```python
from build123d import *

# Parameters (mm, degrees)
BOSS_EXTRUDE1_DEPTH = 0.3
SKETCH2_R           = 0.35
CUT_EXTRUDE1_DEPTH  = 0.3
CUT_EXTRUDE2_DEPTH  = 0.1


with BuildPart() as part:
    # Sketch1 → Boss-Extrude1 (new body)
    with BuildSketch(Plane(origin=(0, 0, 0), x_dir=(1, 0, 0), z_dir=(0, 1, 0))):
        with BuildLine():
            Line((-0.220137797, 1.319636721), (-0.220137797, 0.643381186))
            ThreePointArc((-0.220137797, 0.643381186), (0, -0.68), (0.220137797, 0.643381186))
            Line((0.220137797, 0.643381186), (0.220137797, 1.319636721))
            Line((0.220137797, 1.319636721), (0.34069528, 1.375278636))
            Line((0.34069528, 1.375278636), (0.507155702, 10.530443548))
            Line((0.507155702, 10.530443548), (0, 12))
            Line((0, 12), (-0.507155702, 10.530443548))
            Line((-0.507155702, 10.530443548), (-0.34069528, 1.375278636))
            Line((-0.34069528, 1.375278636), (-0.220137797, 1.319636721))
        make_face()
    extrude(amount=BOSS_EXTRUDE1_DEPTH)

    # Sketch2 → Cut-Extrude1 (cut)
    with BuildSketch(Plane(origin=(0, 0.3, 0), x_dir=(1, 0, 0), z_dir=(0, 1, 0))):
        Circle(SKETCH2_R)
    extrude(amount=-CUT_EXTRUDE1_DEPTH, mode=Mode.SUBTRACT)

    # Sketch3 → Cut-Extrude2 (cut)
    with BuildSketch(Plane(origin=(0, 0.3, 0), x_dir=(1, 0, 0), z_dir=(0, 1, 0))):
        Polygon((0, 11.340864844), (0.303891547, 10.460295461), (0.151945774, 1.527775516), (-0.151945774, 1.527775516), (-0.303891547, 10.460295461), align=None)
    extrude(amount=-CUT_EXTRUDE2_DEPTH, mode=Mode.SUBTRACT)


solid = part.part
```
Part model, mm, in its own coordinate system. Round coordinates to 2 decimals unless told otherwise and drop trailing zeros. Order: outer loops, then holes, each group sorted by start corner. A loop starts at its lowest first (then second) coordinate and runs counter-clockwise, first axis right, second up. Notation, with made-up numbers: M 70,23.5 L 96,23.5 A26 ccw 96,47.5 Z; hole C 52.25,18 d3. An arc over 180 degrees is marked long. Answer in a Markdown table with one row per item. Add a question column.
Q1. Cut at B-B on y = 0.05. Give the cut face in (x, z), and give its area (3 significant figures).
Q2. Cut at C-C on z = -9.5. Give the cut face in (x, y), and give its area (3 significant figures).
Q3. Wall check: L1, parallel to X at y = 0.2, z = 0; L2, parallel to X at y = 0.1, z = 0.25; L3, parallel to Y at x = 0.05, z = -6. Give the ranges that are in metal, low to high. Write a range as from..to.
Q4. Cut at D-D on z = -6.25. Give the cut face in (x, y), and give its area (3 significant figures).
Q5. Cut at A-A on z = 0. Give the cut face in (x, y).
Established:
| question | item | result |
|---|---|---|
| 1 | outline | M -0.51,-10.53 L 0,-12 L 0.51,-10.53 L 0.34,-1.38 L 0.22,-1.32 L 0.22,-0.64 A0.68 ccw long -0.22,-0.64 L -0.22,-1.32 L -0.34,-1.38 Z; hole C 0,0 d0.7 |
| 1 | area | 9.89 mm2 |
| 2 | outline | M -0.49,0 L 0.49,0 L 0.49,0.3 L 0.29,0.3 L 0.29,0.2 L -0.29,0.2 L -0.29,0.3 L -0.49,0.3 Z |
| 2 | area | 0.236 mm2 |
| 3 | L1 | x = -0.68..-0.35, 0.35..0.68 |
| 3 | L2 | x = -0.63..-0.24, 0.24..0.63 |
| 3 | L3 | y = 0..0.2 |
| 4 | outline | M -0.43,0 L 0.43,0 L 0.43,0.3 L 0.23,0.3 L 0.23,0.2 L -0.23,0.2 L -0.23,0.3 L -0.43,0.3 Z |
| 4 | area | 0.211 mm2 |
| 5 | outline | M -0.68,0 L -0.35,0 L -0.35,0.3 L -0.68,0.3 Z; M 0.35,0 L 0.68,0 L 0.68,0.3 L 0.35,0.3 Z |
